```python
from build123d import *

# Parameters (mm, degrees)
F0_R     = 1.3
F0_W     = 38.5
F0_H     = 71
F1_DEPTH = 11.8
F3_DEPTH = 200


with BuildPart() as f1:
    # F0 (on Top) → F1 (new body)
    with BuildSketch(Plane.XY):
        with BuildLine():
            Line((20.5, 45), (-20.5, 45))
            ThreePointArc((-20.5, 45), (-21.914214, 44.414214), (-22.5, 43))
            Line((-22.5, 43), (-22.5, -43))
            ThreePointArc((-22.5, -43), (-21.914214, -44.414214), (-20.5, -45))
            Line((-20.5, -45), (20.5, -45))
            ThreePointArc((20.5, -45), (21.914214, -44.414214), (22.5, -43))
            Line((22.5, -43), (22.5, 43))
            ThreePointArc((22.5, 43), (21.914214, 44.414214), (20.5, 45))
        make_face()
        with Locations((-18.5, -41)):
            Circle(F0_R, mode=Mode.SUBTRACT)
        with Locations((18.5, -41)):
            Circle(F0_R, mode=Mode.SUBTRACT)
        with Locations((-18.5, 41)):
            Circle(F0_R, mode=Mode.SUBTRACT)
        Rectangle(F0_W, F0_H, mode=Mode.SUBTRACT)
        with Locations((18.5, 41)):
            Circle(F0_R, mode=Mode.SUBTRACT)
    extrude(amount=F1_DEPTH)

    # F2 (on Front) → F3 (cut, symmetric)
    with BuildSketch(Plane.XZ):
        Polygon((22.5, 2.122146), (-22.5, 0), (22.5, 0), align=None)
    extrude(amount=F3_DEPTH, both=True, mode=Mode.SUBTRACT)


solid = f1.part
```
The listing builds one solid part. Answer for the finished solid, in the listing's coordinates (mm). A direction names the side the tool comes from. Give positions to 0.01 mm unless a question says otherwise; leave off trailing zeros. Write each loop counter-clockwise with the first axis right and the second up, starting at its lowest first coordinate (ties: lowest second). Pieces come first, ordered by that corner, then holes. Notation, with made-up numbers: M 50,40 L 75,40 A34 cw 75,72 Z; hole C 71,-27.75 d8. An arc over 180 degrees is marked long. Write each question's results on one line, items separated by ' | '.
Q1. Section A-A, the plane y = 18 is taken. Write down the section's boundary in (x, z), then the cut area to 3 significant figures.
Output values:
outline: M -22.5,0 L -19.25,0.15 L -19.25,11.8 L -22.5,11.8 Z; M 19.25,1.97 L 22.5,2.12 L 22.5,11.8 L 19.25,11.8 Z | area: 69.8 mm2
Q2. Section D-D, the plane y = -41 is taken. Write down the section's boundary in (x, z).
Output values:
outline: M -22.5,0 L -19.8,0.13 L -19.8,11.8 L -22.5,11.8 Z; M -17.2,0.25 L 17.2,1.87 L 17.2,11.8 L -17.2,11.8 Z; M 19.8,1.99 L 22.5,2.12 L 22.5,11.8 L 19.8,11.8 Z
Q3. Section C-C, the plane z = 5.75 is taken. Write down the section's boundary in (x, y), then the cut area to 3 significant figures.
Output values:
outline: M -22.5,-43 A2 ccw -20.5,-45 L 20.5,-45 A2 ccw 22.5,-43 L 22.5,43 A2 ccw 20.5,45 L -20.5,45 A2 ccw -22.5,43 Z; hole C -18.5,-41 d2.6; hole C -18.5,41 d2.6; hole M -19.25,-35.5 L 19.25,-35.5 L 19.25,35.5 L -19.25,35.5 Z; hole C 18.5,-41 d2.6; hole C 18.5,41 d2.6 | area: 1,290 mm2
Q4. A tool of negligible diameter and unlimited length cuts with its end or side. For faces 4 (the flat face through (-22.5, 1, 6)), 5 (the flat face through (0, 35.5, 6)), from which of +Z, -Z, +X, -X, +Y, -Y can it reach the whole face along a straight path? Write none if from no direction.
Output values:
face 4: +Z, -Z, -X, +Y, -Y | face 5: +Z, -Z
Q5. Consider L1, parallel to Y at x = -18.5, z = 3; L2, parallel to X at y = -41, z = 8; L3, parallel to Y at x = 14.5, z = 3. Determine where each line is inside the solid, lowest interval first. Write a range as from..to.
Output values:
L1: -45..-42.3, -39.7..-35.5, 35.5..39.7, 42.3..45 | L2: -22.5..-19.8, -17.2..17.2, 19.8..22.5 | L3: -45..-35.5, 35.5..45
Q6. For a pull along Y with two mould halves and no side action, classify faces 1 (the flat face through (0, -45, 6)), 2 (the flat face through (20.32, -0.63, 2.02)), 3 (the flat face through (-19.25, 0, 6)) as released by +Y, released by -Y, zero draft, split by the parting line, or undercut.
Output values:
face 1: released by -Y | face 2: zero draft | face 3: undercut
Q7. A flat-ended cylindrical pin translates along its axis: P1, Ø3, axis at x = 18.5, y = 41, coming from the -Z side. Find the tip coordinate at first contact, or state that the pin passes through.
Output values:
P1: z = 1.86
Q8. Section B-B, the plane x = -15.5 is taken. Write down the section's boundary in (y, z).
Output values:
outline: M -45,0.33 L -35.5,0.33 L -35.5,11.8 L -45,11.8 Z; M 35.5,0.33 L 45,0.33 L 45,11.8 L 35.5,11.8 Z
